Geometry check sheet. Reference: the model listing, model coordinates, mm. A direction names the side the tool comes from. Round coordinates to 2 decimals unless told otherwise and drop trailing zeros. Order: outer loops, then holes, each group sorted by start corner. A loop starts at its lowest first (then second) coordinate and runs counter-clockwise, first axis right, second up. Notation, with made-up numbers: (-36.5, 73) - (-32.5, 73) arc R21 ccw to (-32.5, 112) - close; hole circle Ø5 at (-10, 84). An arc over 180 degrees is marked (long way). Use a Markdown table: item, result. Add a question column.
(1) Mould release check, pull along Z, two halves, no side actions. Record for faces 1 (the face through (2, 26, 0)), 2 (the face through (0, 35, 123)), 3 (the face through (1.12, 41.22, 213.71)): released by +Z, released by -Z, zero draft, split by the parting line, or undercut.
(2) Thickness scan on line 1 along X through (y, z) = (9.5, 29.5). Record the ranges inside material, lowest first. Write a range as [from, to].
(3) Section check A-A on z = 149.5. Record the boundary of the cut face in (x, y), then the cut area to 3 significant figures.
(4) Gauge pin test, flat ends, axial feed: P1, Ø5, axis at x = 22.5, z = 110.5, coming from the -Y side; P2, Ø15, axis at x = 21, z = 156, coming from the +Y side; P3, Ø4, axis at y = 48, z = 111.5, coming from the +X side. Record the tip position at first contact, or that the pin passes through.
(5) Access from +Z, -Z, +X, -X, +Y, -Y to the whole of each face (thin tool, end or side, straight path). Record for faces 4 (the face through (2, 26, 250)), 5 (the face through (3, 38, 123)).
(6) Section check B-B on y = 65. Record the boundary of the cut face in (x, z).
```python
from build123d import *

# Parameters (mm, degrees)
BOSS_EXTRUDE1_DEPTH = 250


# Read off the part's stored shape, not the designer's step: Cavity1
with BuildPart() as part:
    # Sketch1 → Boss-Extrude1 (new body)
    with BuildSketch(Plane.XY):
        Polygon((0, 72), (3, 72), (3, 3), (33, 3), (33, 0), (0, 0), align=None)
    extrude(amount=BOSS_EXTRUDE1_DEPTH)

    # Cavity1 outline → Cavity1 (revolve, cut)
    with BuildSketch(Plane(origin=(0, 43.176202168, 198.837075549), x_dir=(0, 1, 0), z_dir=(0, 0, -1))):
        with BuildLine():
            Line((15, 0), (15, 2.2))
            Line((15, 2.2), (14, 2.2))
            ThreePointArc((14, 2.2), (13.765685425, 2.765685425), (13.2, 3))
            Line((13.2, 3), (0, 3))
            Line((0, 3), (0, 0))
            Line((0, 0), (15, 0))
        make_face()
    revolve(axis=Axis((0, 43.176202168, 198.837075549), (1, 0, 0)), mode=Mode.SUBTRACT)


solid = part.part
```
Check sheet entries:
| question | item | result |
|---|---|---|
| 1 | face 1 | released by -Z |
| 1 | face 2 | zero draft |
| 1 | face 3 | undercut |
| 2 | line 1 | x = [0, 3] |
| 3 | outline | (0, 0) - (33, 0) - (33, 3) - (3, 3) - (3, 72) - (0, 72) - close |
| 3 | area | 306 mm2 |
| 4 | P1 | stops at y = 0 |
| 4 | P2 | stops at y = 3 |
| 4 | P3 | stops at x = 3 |
| 5 | face 4 | +Z, +X, -X, +Y, -Y |
| 5 | face 5 | +Z, -Z, +X, +Y |
| 6 | outline | (0, 0) - (3, 0) - (3, 250) - (0, 250) - close |
